Work out the finished part from the listing and answer in its coordinate system (mm). Face numbers are marked on the shaded views. A direction names the side the tool comes from. Round coordinates to 2 decimals unless told otherwise and drop trailing zeros. Write each loop counter-clockwise with the first axis right and the second up, starting at its lowest first coordinate (ties: lowest second). Pieces come first, ordered by that corner, then holes. Notation, with made-up numbers: (46, 88) -> (67, 88) arc R17 ccw to (67, 104) -> close; hole circle Ø3 at (-31, 15.25). An arc over 180 degrees is marked (long way). One line per item, written item: value.
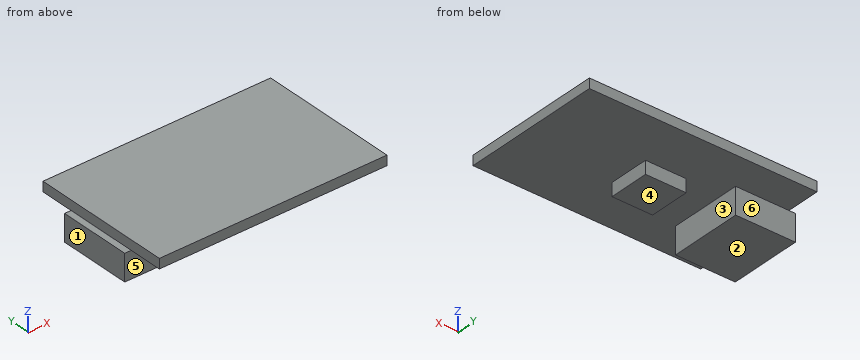
```python
from build123d import *

# Parameters (mm, degrees)
PCB_SK1_W   = 28
PCB_SK1_H   = 17.3
PCB_DEPTH   = 1.2
USB_C_SK2_W = 7.35
USB_C_SK2_H = 8.94
USB_C_DEPTH = 3.26
CHIP_SK3_W  = 5
CHIP_SK3_H  = 5
CHIP_DEPTH  = 1.6


with BuildPart() as part:
    # PCB_Sk1 → PCB (new body)
    with BuildSketch(Plane.XY.offset(-3.17)):
        with Locations((-33.2, -18.55)):
            Rectangle(PCB_SK1_W, PCB_SK1_H)
    extrude(amount=-PCB_DEPTH)

    # USB_C_Sk2 → USB_C (add)
    with BuildSketch(Plane.XY.offset(-4.37)):
        with Locations((-44.325, -18.55)):
            Rectangle(USB_C_SK2_W, USB_C_SK2_H)
    extrude(amount=-USB_C_DEPTH)

    # Chip_Sk3 → Chip (add)
    with BuildSketch(Plane.XY.offset(-4.37)):
        with Locations((-33.7, -18.55)):
            Rectangle(CHIP_SK3_W, CHIP_SK3_H)
    extrude(amount=-CHIP_DEPTH)


solid = part.part
```
(1) For a pull along X with two mould halves and no side action, classify the marked faces 1, 2 and 3 as pulls with the +X half, pulls with the -X half, needs draft (parallel to the pull), parting line crosses it, or undercut.
Reported:
face 1: pulls with the -X half
face 2: needs draft
face 3: undercut
(2) A tool of negligible diameter and unlimited length cuts with its end or side. For the marked faces 4, 5 and 6, from which of +Z, -Z, +X, -X, +Y, -Y can it reach the whole face along a straight path? Write none if from no direction.
Reported:
face 4: -Z, +X, +Y, -Y
face 5: -Z, +X, -X, -Y
face 6: -Z, +X, -X, +Y
(3) Find section A-A on z = -5.35. Give the vertices of the cut face in (x, y), plus the area to 3 significant figures.
Reported:
outline: (-48, -23.02) -> (-40.65, -23.02) -> (-40.65, -14.08) -> (-48, -14.08) -> close; (-36.2, -21.05) -> (-31.2, -21.05) -> (-31.2, -16.05) -> (-36.2, -16.05) -> close
area: 90.7 mm2
(4) Flat-ended cylindrical pins translate along their axes: pin 1 Ø2.5 at (x, z) = (-46, -5.5) entering from -Y; pin 2 Ø1.5 at (y, z) = (-16, -5.5) entering from +X; pin 3 Ø2.5 at (x, z) = (-43.5, -6.5) entering from +Y; pin 4 Ø0.8 at (x, z) = (-33.5, -5) entering from -Y. Find the tip coordinate at first contact, or state that the pin passes through.
Reported:
pin 1: stops at y = -27.2
pin 2: stops at x = -31.2
pin 3: stops at y = -14.08
pin 4: stops at y = -21.05
(5) Find section B-B on x = -32. Give the vertices of the cut face in (y, z), plus the area to 3 significant figures.
Reported:
outline: (-27.2, -4.37) -> (-21.05, -4.37) -> (-21.05, -5.97) -> (-16.05, -5.97) -> (-16.05, -4.37) -> (-9.9, -4.37) -> (-9.9, -3.17) -> (-27.2, -3.17) -> close
area: 28.8 mm2
(6) Find section C-C on y = -14.5. Give the vertices of the cut face in (x, z), plus the area to 3 significant figures.
Reported:
outline: (-48, -7.63) -> (-40.65, -7.63) -> (-40.65, -4.37) -> (-19.2, -4.37) -> (-19.2, -3.17) -> (-47.2, -3.17) -> (-47.2, -4.37) -> (-48, -4.37) -> close
area: 57.6 mm2
(7) Consider probe 1 along X at (y, z) = (-16.75, -5.65); probe 2 along Y at (x, z) = (-41, -6.05); probe 3 along Z at (x, y) = (-25.25, -17.25). Determine where each line is inside the solid, lowest interval first.
Reported:
probe 1: x = -48 to -40.65, -36.2 to -31.2
probe 2: y = -23.02 to -14.08
probe 3: z = -4.37 to -3.17
(8) Find section D-D on z = -3.6. Give the vertices of the cut face in (x, y).
Reported:
outline: (-47.2, -27.2) -> (-19.2, -27.2) -> (-19.2, -9.9) -> (-47.2, -9.9) -> close
